The model under review builds one solid part; all positions refer to its coordinate system, in mm. A direction names the side the tool comes from. Coordinates: 2 decimals unless noted, no trailing zeros. Loops run counter-clockwise (first coordinate to the right, second up) from the corner with the lowest first, then second, coordinate; pieces in that order, holes last. Notation, with made-up numbers: (79, -29.75) - (97, -29.75) arc R29 cw to (97, -7.75) - close; hole circle Ø5 at (-11.75, 52.25). An arc over 180 degrees is marked (long way). Answer in a Markdown table with one row per item. Add a question column.
(1) For line 1 along Z through (x, y) = (-39, -3.25); line 2 along Z through (x, y) = (0, -4.5); line 3 along Z through (x, y) = (28, -7.75), list the stretches that pass through material, from the lowest coordinate up.
(2) For P1, Ø3.5, axis at x = 42, y = -7, coming from the -Z side; P2, Ø4, axis at y = -3.5, z = -22, coming from the -X side; P3, Ø3.5, axis at x = -41, y = -6, coming from the -Z side, all flat-tipped, find the tip position at first contact; note any pin that passes through.
(3) We need section B-B on z = 25. Write out the cut boundary in (x, y).
(4) Mouldability with a two-part tool opening along Z and no side actions: class faces 1 (the cylindrical face through (-27, -7, -25)), 2 (the cylindrical face through (43.289, -7.098, 38.196)), 3 (the flat face through (-45, -7, 0)) as +Z half, -Z half, draft (parallel to the pull), parting line (faces both ways), or undercut.
(5) We need section A-A on x = 0. Write out the cut boundary in (y, z).
(6) We need section D-D on z = -25. Write out the cut boundary in (x, y).
(7) Machinability: for faces 4 (the flat face through (39, -7, 19)), 5 (the flat face through (45, -7, 32)), 6 (the flat face through (-39, -7, -19)), which of the approach directions +Z, -Z, +X, -X, +Y, -Y give a long, thin tool a straight path to every point of the face, cutting with its end or side? Answer none if there is none.
(8) We need section C-C on y = -5.5. Write out the cut boundary in (x, z), plus the area to 3 significant figures.
from build123d import *

# Parameters (mm, degrees)
F1_DEPTH = 14
F2_R     = 6
F4_D     = 11


with BuildPart() as f1:
    # F0 (on Front) → F1 (new body)
    with BuildSketch(Plane.XZ):
        with BuildLine():
            Line((45, 31), (45, 40))
            Line((45, 40), (-45, 40))
            Line((-45, 40), (-45, 31))
            Line((-45, 31), (-33, 31))
            ThreePointArc((-33, 31), (-27, 25), (-33, 19))
            Line((-33, 19), (-45, 19))
            Line((-45, 19), (-45, -19))
            Line((-45, -19), (-33, -19))
            ThreePointArc((-33, -19), (-27, -25), (-33, -31))
            Line((-33, -31), (-45, -31))
            Line((-45, -31), (-45, -40))
            Line((-45, -40), (45, -40))
            Line((45, -40), (45, -31))
            Line((45, -31), (33, -31))
            ThreePointArc((33, -31), (27, -25), (33, -19))
            Line((33, -19), (45, -19))
            Line((45, -19), (45, 19))
            Line((45, 19), (33, 19))
            ThreePointArc((33, 19), (27, 25), (33, 31))
            Line((33, 31), (45, 31))
        make_face()
    extrude(amount=F1_DEPTH)

    # F2
    f2_edges = [f1.edges().sort_by_distance(p)[0] for p in [
        (-45, -7, 40),
        (-45, -7, -40),
        (45, -7, 40),
        (45, -7, -40),
    ]]
    fillet(f2_edges, radius=F2_R)

    # F4 (through all)
    with Locations(Plane.XZ.offset(14)):
        with Locations((0, 25)):
            Hole(F4_D / 2)


solid = f1.part
Outcome:
| question | item | result |
|---|---|---|
| 1 | line 1 | -40 to -31, -19 to 19, 31 to 40 |
| 1 | line 2 | -40 to 19.5, 30.5 to 40 |
| 1 | line 3 | -40 to -28.32, -21.68 to 21.68, 28.32 to 40 |
| 2 | P1 | z = -39.87 |
| 2 | P2 | x = -29.68 |
| 2 | P3 | z = -39.99 |
| 3 | outline | (-27, -14) - (-5.5, -14) - (-5.5, 0) - (-27, 0) - close; (5.5, -14) - (27, -14) - (27, 0) - (5.5, 0) - close |
| 4 | face 1 | undercut |
| 4 | face 2 | +Z half |
| 4 | face 3 | draft |
| 5 | outline | (-14, -40) - (0, -40) - (0, 19.5) - (-14, 19.5) - close; (-14, 30.5) - (0, 30.5) - (0, 40) - (-14, 40) - close |
| 6 | outline | (-27, -14) - (27, -14) - (27, 0) - (-27, 0) - close |
| 7 | face 4 | +X, +Y, -Y |
| 7 | face 5 | +Z, -Z, +X, +Y, -Y |
| 7 | face 6 | -X, +Y, -Y |
| 8 | outline | (-45, -34) arc R6 ccw to (-39, -40) - (39, -40) arc R6 ccw to (45, -34) - (45, -31) - (33, -31) arc R6 cw to (33, -19) - (45, -19) - (45, 19) - (33, 19) arc R6 cw to (33, 31) - (45, 31) - (45, 34) arc R6 ccw to (39, 40) - (-39, 40) arc R6 ccw to (-45, 34) - (-45, 31) - (-33, 31) arc R6 cw to (-33, 19) - (-45, 19) - (-45, -19) - (-33, -19) arc R6 cw to (-33, -31) - (-45, -31) - close; hole circle Ø11 at (0, 25) |
| 8 | area | 6,270 mm² |
